```python
from build123d import *

# Parameters (mm, degrees)
SZKIC1_W                                          = 230
SZKIC1_H                                          = 150
DODANIE_WYCI_GNI_CIE1_DEPTH                       = 5
POG_BIENIE_WALCOWE_POD_M3_RUB_Z_BEM_S_D           = 3.6
POG_BIENIE_WALCOWE_POD_M3_RUB_Z_BEM_S_DEPTH       = 6.7
POG_BIENIE_WALCOWE_POD_M3_RUB_Z_BEM_S_CBORE_D     = 7
POG_BIENIE_WALCOWE_POD_M3_RUB_Z_BEM_S_CBORE_DEPTH = 2.4
POG_BIENIE_WALCOWE_POD_M3_RUB_Z_BEM_S_TIP         = 1.081549114


with BuildPart() as part:
    # Szkic1 → Dodanie-wyciągnięcie1 (new body)
    with BuildSketch(Plane.XY):
        Rectangle(SZKIC1_W, SZKIC1_H)
    extrude(amount=DODANIE_WYCI_GNI_CIE1_DEPTH)

    # Pogłębienie walcowe pod M3 Śrubę z łbem stożkowym ściętym1
    with Locations(Plane(origin=(0, 0, 0), x_dir=(-1, 0, 0), z_dir=(0, 0, -1))):
        with Locations((105, 37.5), (105, 0), (105, -37.5), (-105, -37.5), (-105, 0), (-105, 37.5)):
            CounterBoreHole(POG_BIENIE_WALCOWE_POD_M3_RUB_Z_BEM_S_D / 2, POG_BIENIE_WALCOWE_POD_M3_RUB_Z_BEM_S_CBORE_D / 2, POG_BIENIE_WALCOWE_POD_M3_RUB_Z_BEM_S_CBORE_DEPTH, depth=POG_BIENIE_WALCOWE_POD_M3_RUB_Z_BEM_S_DEPTH)
            with Locations((0, 0, -(POG_BIENIE_WALCOWE_POD_M3_RUB_Z_BEM_S_DEPTH + POG_BIENIE_WALCOWE_POD_M3_RUB_Z_BEM_S_TIP / 2))):  # 118° drill point
                Cone(0, POG_BIENIE_WALCOWE_POD_M3_RUB_Z_BEM_S_D / 2, POG_BIENIE_WALCOWE_POD_M3_RUB_Z_BEM_S_TIP, mode=Mode.SUBTRACT)


solid = part.part
```
Work out the finished part from the listing and answer in its coordinate system (mm). A direction names the side the tool comes from. Give positions to 0.01 mm unless a question says otherwise; leave off trailing zeros. Put each result on its own line as item: value. Start each with the question number.
Item 1: This flat-tipped pin is pushed along its axis until it touches: P1, Ø5.5, axis at x = 105, y = 37.5, coming from the -Z side. Where does it stop, or does it pass through?
Item 2: The mould has two halves that part along X. Classify faces 3 (the face through (101.66, 38.55, 1.18)), 4 (the face through (-2, 75, 2)), 5 (the face through (-108.233, -1.341, 1.183)), 6 (the face through (115, -1, 2)): released by +X, released by -X, zero draft, split by the parting line, or undercut.
Item 3: Which of the six approach directions +Z, -Z, +X, -X, +Y, -Y give full straight-line access (tool end or side, diameter ignored) to faces 1 (the face through (-2, 1, 5)), 2 (the face through (-108.34, -36.45, 1.18))?
Item 4: Find the intervals of material crossed by L1, parallel to Y at x = -105, z = 3.5; L2, parallel to Y at x = -105, z = 1.1; L3, parallel to X at y = 36, z = 3.3, in increasing order. Write a range as [from, to].
Answers below:
1. P1: z = 2.4
2. face 3: undercut
2. face 4: zero draft
2. face 5: undercut
2. face 6: released by +X
3. face 1: +Z, +X, -X, +Y, -Y
3. face 2: -Z
4. L1: [-75, -39.3], [-35.7, -1.8], [1.8, 35.7], [39.3, 75]
4. L2: [-75, -41], [-34, -3.5], [3.5, 34], [41, 75]
4. L3: [-115, -105.99], [-104.01, 104.01], [105.99, 115]
